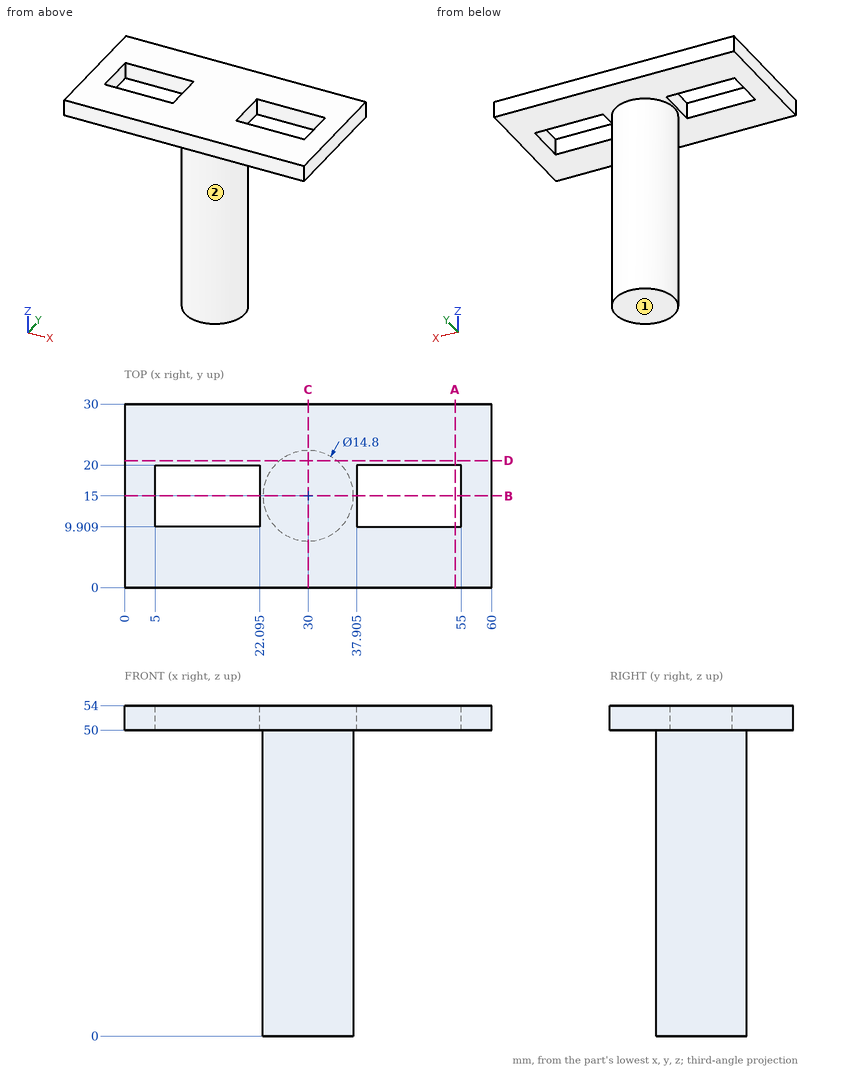
Here's the drawing with two shaded views (mm, measured from the low corner). I have some questions. A direction names the side the tool comes from. Give positions to 0.01 mm unless a question says otherwise; leave off trailing zeros. Loops run counter-clockwise (first coordinate to the right, second up) from the corner with the lowest first, then second, coordinate; pieces in that order, holes last. Notation, with made-up numbers: M -34,18.25 L 13,18.25 A21 ccw 13,24.25 Z; hole C 28,-13 d4. An arc over 180 degrees is marked long. Use one line per item in the form item = value. Start each with the question number.
(1) I want a section at B-B, the plane y = 15. Write out the boundary of the cut face in (x, z) (1 decimal), and give its area (3 significant figures).
(2) On a 3-axis mill with a long thin cutter (end or side, diameter ignored), from which of +Z, -Z, +X, -X, +Y, -Y can I reach the whole of each face in a straight line? I mean the marked faces 1 and 2. Say none if no direction works.
(3) I'm going to push flat-ended pins straight in: P1, Ø8, axis at x = 32.5, z = 20.5, coming from the -Y side; P2, Ø1, axis at y = 21, z = 10.5, coming from the -X side; P3, Ø4, axis at y = 21, z = 21.5, coming from the +X side (1 decimal); P4, Ø8, axis at x = 44.5, z = 12.5, coming from the +Y side. Where does each tip first touch, or does it pass through?
(4) I want a section at A-A, the plane x = 54. Write out the boundary of the cut face in (y, z).
(5) I want a section at C-C, the plane x = 30. Write out the boundary of the cut face in (y, z).
(6) I want a section at D-D, the plane y = 20.75. Write out the boundary of the cut face in (x, z), and give its area (3 significant figures).
(7) Please list where these lines run through material, in increasing order: line 1 (X direction, y = 14, z = 52) (1 decimal); line 2 (Z direction, x = 7.5, y = 26.75); line 3 (Y direction, x = 30, z = 6).
Worked out:
q1.outline = M 0,50 L 5,50 L 5,54 L 0,54 Z; M 22.1,50 L 22.6,50 L 22.6,0 L 37.4,0 L 37.4,50 L 37.9,50 L 37.9,54 L 22.1,54 Z; M 55,50 L 60,50 L 60,54 L 55,54 Z
q1.area = 843 mm²
q2.face_1 = -Z, +X, -X, +Y, -Y
q2.face_2 = -Z
q3.P1 = 7.6
q3.P2 = 25.05
q3.P3 = 36.2
q3.P4 = through
q4.outline = M 0,50 L 9.91,50 L 9.91,54 L 0,54 Z; M 20,50 L 30,50 L 30,54 L 20,54 Z
q5.outline = M 0,50 L 7.6,50 L 7.6,0 L 22.4,0 L 22.4,50 L 30,50 L 30,54 L 0,54 Z
q6.outline = M 0,50 L 25.34,50 L 25.34,0 L 34.66,0 L 34.66,50 L 60,50 L 60,54 L 0,54 Z
q6.area = 706 mm²
q7.line_1 = 0 to 5, 22.1 to 37.9, 55 to 60
q7.line_2 = 50 to 54
q7.line_3 = 7.6 to 22.4
